from build123d import *

# Parameters (mm, degrees)
SKETCH1_W                 = 25.4
SKETCH1_H                 = 63.5
SKETCH1_H_2               = 12.7
BOSS_EXTRUDE1_DEPTH       = 160.782
CUT_EXTRUDE2_DEPTH        = 168.175421411
CUT_EXTRUDE2_DEPTH_BACK   = 168.175421411
BOSS_EXTRUDE2_REACH       = 177.247
SKETCH1_5_W               = 25.4
SKETCH1_5_H               = 12.7
SKETCH8_W                 = 25.4
SKETCH8_H                 = 3.175
BOSS_EXTRUDE3_DEPTH       = 12.7
FILLET1_R                 = 6.35
BOSS_EXTRUDE4_START       = -162.209174004
BOSS_EXTRUDE4_OUTLINE_R   = 5.08
BOSS_EXTRUDE4_DEPTH       = 17.209174004
BOSS_EXTRUDE4_START_2     = 162.209174004
BOSS_EXTRUDE4_2_OUTLINE_R = 5.08
BOSS_EXTRUDE4_2_DEPTH     = 3.399488646
BOSS_EXTRUDE4_START_3     = 155.438704549
BOSS_EXTRUDE4_3_OUTLINE_W = 14
BOSS_EXTRUDE4_3_OUTLINE_H = 14
BOSS_EXTRUDE4_3_DEPTH     = 4.561295451
CUT_EXTRUDE5_START        = -15.875
SKETCH9_3_R               = 5.715
SKETCH9_3_R_2             = 5.08
CUT_EXTRUDE5_DEPTH        = 15.875


with BuildPart() as part:
    # Sketch1 → Boss-Extrude1 (new body)
    with BuildSketch(Plane(origin=(0, 0, 0), x_dir=(1, 0, 0), z_dir=(0, 1, 0))):
        with Locations((0, -6.35)):
            Rectangle(SKETCH1_W, SKETCH1_H)
        with Locations((0, 31.75)):
            Rectangle(SKETCH1_W, SKETCH1_H_2)
    extrude(amount=BOSS_EXTRUDE1_DEPTH)

    # Sketch4 → Cut-Extrude2 (cut, two sides: drawn at the far end of the back side and taken through both)
    with BuildSketch(Plane(origin=(12.7, 0, 0), x_dir=(0, 0, -1), z_dir=(1, 0, 0)).offset(-CUT_EXTRUDE2_DEPTH_BACK)):
        Polygon((38.1, 160.782), (-38.1, 160.782), (-38.1, 135.285836654), align=None)
    extrude(amount=CUT_EXTRUDE2_DEPTH + CUT_EXTRUDE2_DEPTH_BACK, mode=Mode.SUBTRACT)

    # Boss-Extrude2: from a plane face, 177.247 long prism both ways, kept between that surface and its translate by the depth
    boss_extrude2_start = Plane(origin=(-12.7, 135.285836654, 38.1), z_dir=(0, -0.9483236552061991, -0.31730465640509276)) * Box(710.988, 710.988, 355.494, align=(Align.CENTER, Align.CENTER, Align.MIN), mode=Mode.PRIVATE)
    boss_extrude2_end = Plane(origin=(-12.7, 144.810836654, 38.1), z_dir=(0, -0.9483236552061991, -0.31730465640509276)) * Box(710.988, 710.988, 355.494, align=(Align.CENTER, Align.CENTER, Align.MIN), mode=Mode.PRIVATE)
    # Sketch1_5 → Boss-Extrude2 (add, from a surface)
    with BuildSketch(Plane(origin=(0, 0, 0), x_dir=(1, 0, 0), z_dir=(0, 1, 0)), mode=Mode.PRIVATE) as boss_extrude2_sk1:
        with Locations((0, 31.75)):
            Rectangle(SKETCH1_5_W, SKETCH1_5_H)
    boss_extrude2_tool1 = extrude(boss_extrude2_sk1.sketch, amount=BOSS_EXTRUDE2_REACH, both=True, mode=Mode.PRIVATE)
    add(((boss_extrude2_tool1 - boss_extrude2_start) & boss_extrude2_end).solids().sort_by_distance((0, 161.295139, -31.75))[0])

    # Sketch8 → Boss-Extrude3 (add, along a direction that is not the sketch's normal)
    with BuildSketch(Plane.XY.offset(-25.4)):
        with Locations((0, 164.470139442)):
            Rectangle(SKETCH8_W, SKETCH8_H)
    extrude(amount=BOSS_EXTRUDE3_DEPTH, dir=(0, -0.31730465640509276, 0.9483236552061991))

    # Fillet1
    fillet1_edges = [part.edges().sort_by_distance(p)[0] for p in [
        (-12.7, 67.642918327, 38.1),
        (12.7, 67.642918327, 38.1),
        (-12.7, 85.1535, -38.1),
        (12.7, 85.1535, -38.1),
    ]]
    fillet(fillet1_edges, radius=FILLET1_R)

    # Boss-Extrude4: read off the stored shape, not the designer's step
    # Boss-Extrude4 outline → Boss-Extrude4 (add)
    with BuildSketch(Plane.XZ.offset(BOSS_EXTRUDE4_START)):
        Circle(BOSS_EXTRUDE4_OUTLINE_R)
    extrude(amount=BOSS_EXTRUDE4_DEPTH)

    # Boss-Extrude4 2 outline → Boss-Extrude4 2 (add)
    with BuildSketch(Plane(origin=(0, 0, 0), x_dir=(1, 0, 0), z_dir=(0, 1, 0)).offset(BOSS_EXTRUDE4_START_2)):
        Circle(BOSS_EXTRUDE4_2_OUTLINE_R)
    extrude(amount=BOSS_EXTRUDE4_2_DEPTH)

    # Boss-Extrude4 3 outline → Boss-Extrude4 3 (cut)
    with BuildSketch(Plane(origin=(0, 0, 0), x_dir=(1, 0, 0), z_dir=(0, 0.9483236552061991, 0.31730465640509303)).offset(BOSS_EXTRUDE4_START_3)):
        with Locations((0, 52)):
            Rectangle(BOSS_EXTRUDE4_3_OUTLINE_W, BOSS_EXTRUDE4_3_OUTLINE_H)
    extrude(amount=BOSS_EXTRUDE4_3_DEPTH, mode=Mode.SUBTRACT)

    # Sketch9_3 → Cut-Extrude5 (cut)
    # profile 1 of 2: a face of its own
    with BuildSketch(Plane.XZ.offset(CUT_EXTRUDE5_START)):
        with Locations(Location((0, 0, 0), (0, 0, 270))):
            Circle(SKETCH9_3_R)
        with Locations(Location((0, 0, 0), (0, 0, 90))):
            Circle(SKETCH9_3_R_2, mode=Mode.SUBTRACT)
    # profile 2 of 2: a face of its own
    with BuildSketch(Plane.XZ.offset(CUT_EXTRUDE5_START)):
        with Locations(Location((0, 0, 0), (0, 0, 90))):
            Circle(SKETCH9_3_R_2)
    extrude(amount=CUT_EXTRUDE5_DEPTH, mode=Mode.SUBTRACT)


solid = part.part
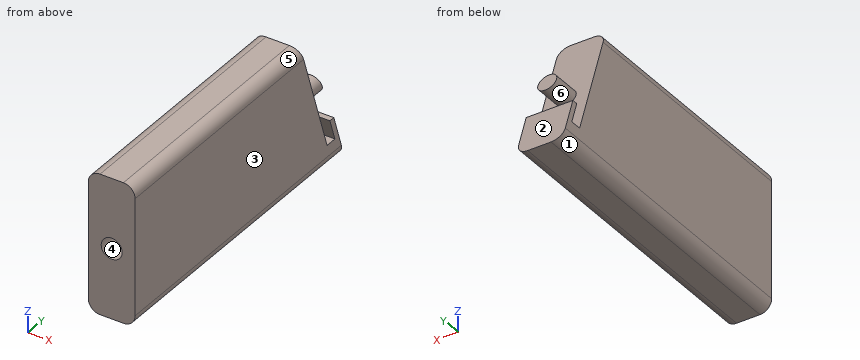
Could you check a few things on this model? Use its own coordinates, in mm. Face numbers are marked on the shaded views. A direction names the side the tool comes from. Give positions to 0.01 mm unless a question says otherwise; leave off trailing zeros. Order: outer loops, then holes, each group sorted by start corner. A loop starts at its lowest first (then second) coordinate and runs counter-clockwise, first axis right, second up. Notation, with made-up numbers: (39, -11.75) -> (97, -11.75) arc R34 ccw to (97, 26.25) -> close; hole circle Ø11 at (9, 30). An arc over 180 degrees is marked (long way). Answer in a Markdown table with one row per item. Add a question column.
Item 1: Imagine slicing it at C-C (x = -8.5). List the corners of the cut face in (y, z) for me.
Item 2: I'm going to push flat-ended pins straight in: P1, Ø1.9, axis at x = 0, y = 160.5, coming from the +Z side; P2, Ø9, axis at x = 0, z = 0, coming from the +Y side; P3, Ø1, axis at x = 9, z = -25, coming from the +Y side. Where does each tip first touch, or does it pass through?
Item 3: Imagine slicing it at B-B (z = -19). List the corners of the cut face in (x, y) for me, and give its area (3 significant figures).
Item 4: Imagine slicing it at A-A (y = 52). List the corners of the cut face in (x, z) for me, and give its area (3 significant figures).
Item 5: For the marked faces 5 and 6, which set-ups out of +Z, -Z, +X, -X, +Y, -Y let a thin tool reach every point of the face, with its end or its side?
Item 6: Please list where these lines run through material, in increasing order: probe 1 along X at (y, z) = (6, 0) (3 decimals); probe 2 along Y at (x, z) = (-3, -13.5); probe 3 along Y at (x, z) = (0, -28).
Item 7: We'd pull the mould along Z, two halves only. Please class the marked faces 1, 2, 3 and 4: pulls with the +Z half, pulls with the -Z half, needs draft (parallel to the pull), parting line crosses it, or undercut.
Item 8: Imagine slicing it at D-D (z = 0). List the corners of the cut face in (x, y) for me (3 decimals).
Result:
| question | item | result |
|---|---|---|
| 1 | outline | (0, -37.72) -> (170.18, -37.72) -> (162.03, -13.36) -> (158.85, -13.36) -> (162.88, -25.4) -> (156.53, -25.4) -> (135.41, 37.72) -> (0, 37.72) -> close |
| 2 | P1 | z = 5.08 |
| 2 | P2 | y = 165.41 |
| 2 | P3 | y = 166.09 |
| 3 | outline | (-12.7, 0) -> (12.7, 0) -> (12.7, 154.39) -> (-12.7, 154.39) -> close; (-12.7, 160.74) -> (12.7, 160.74) -> (12.7, 163.92) -> (-12.7, 163.92) -> close |
| 3 | area | 4,000 mm2 |
| 4 | outline | (-12.7, -31.75) arc R6.35 ccw to (-6.35, -38.1) -> (6.35, -38.1) arc R6.35 ccw to (12.7, -31.75) -> (12.7, 31.75) arc R6.35 ccw to (6.35, 38.1) -> (-6.35, 38.1) arc R6.35 ccw to (-12.7, 31.75) -> close |
| 4 | area | 1,900 mm2 |
| 5 | face 5 | +Z, +X, +Y, -Y |
| 5 | face 6 | +Y |
| 6 | probe 1 | -12.7 to -5.715, 5.715 to 12.7 |
| 6 | probe 2 | 0 to 152.55, 158.9 to 162.08 |
| 6 | probe 3 | 0 to 166.93 |
| 7 | face 1 | pulls with the -Z half |
| 7 | face 2 | undercut |
| 7 | face 3 | needs draft |
| 7 | face 4 | undercut |
| 8 | outline | (-12.7, 0) -> (-5.715, 0) -> (-5.715, 15.875) -> (5.715, 15.875) -> (5.715, 0) -> (12.7, 0) -> (12.7, 148.034) -> (5.08, 148.034) -> (5.08, 163.909) -> (-5.08, 163.909) -> (-5.08, 148.034) -> (-12.7, 148.034) -> close |
